Autodesk Inventor part; units mm, degrees
ref_plane "YZ Plane" through (0, 0, 0) normal (1, 0, 0) x (0, 1, 0)
ref_plane "XZ Plane" through (0, 0, 0) normal (0, 1, 0) x (-1, 0, 0)
ref_plane "XY Plane" through (0, 0, 0) normal (0, 0, 1) x (1, 0, 0)
sketch "スケッチ1" plane through (0, 0, 0) normal (0, 0, 1) x (1, 0, 0)
  circle A0 centre (0, 0) radius 1.5
  dimension "d0" = 3
extrude "押し出し1" add sketch "スケッチ1" along normal blind 6
sketch "スケッチ2" plane through (0, 0, 6) normal (0, 0, 1) x (1, 0, 0)
  circle A0 centre (0, 0) radius 1.5
  circle A1 centre (0, 0) radius 3
  dimension "d3" = 6
extrude "押し出し2" add sketch "スケッチ2" along normal blind 2 contours A0 | A1
fillet "フィレット1" radius 2 1 edges at (-3, 0, 8)
thread "ねじ1"
sketch "スケッチ3" plane through (0, 0, 0) normal (0, 0, -1) x (-1, 0, 0)
  circle A0 centre (0, 0) radius 1.5
extrude "押し出し3" add sketch "スケッチ3" along normal blind 9
sketch "スケッチ4" plane through (0, 0, 8) normal (0, 0, 1) x (1, 0, 0)
  line L0 (0.8191, 1.1885) -> (1.4388, -0.1151)
  line L1 (1.4388, -0.1151) -> (0.6197, -1.3036)
  line L2 (0.6197, -1.3036) -> (-0.8191, -1.1885)
  line L3 (-0.8191, -1.1885) -> (-1.4388, 0.1151)
  line L4 (-1.4388, 0.1151) -> (-0.6197, 1.3036)
  line L5 (-0.6197, 1.3036) -> (0.8191, 1.1885)
  point P0 (0, 0)
  point P1 (0, 0)
  dimension "d11" = 2.5
extrude "押し出し4" cut sketch "スケッチ4" against normal blind 1.3
properties part number "SB　15mmなべネジ" material "Steel, Mild"
The listing builds one solid part. Answer for the finished solid, in the listing's coordinates (mm). A direction names the side the tool comes from. Round coordinates to 2 decimals unless told otherwise and drop trailing zeros. Write each loop counter-clockwise with the first axis right and the second up, starting at its lowest first coordinate (ties: lowest second). Pieces come first, ordered by that corner, then holes. Notation, with made-up numbers: M -14.75,71 L -1.75,71 A16 ccw -1.75,89 Z; hole C 32.5,41 d10. An arc over 180 degrees is marked long. Write each question's results on one line, items separated by ' | '. Start each with the question number.
Item 1: A cutting plane is placed at A-A on z = -5. Write down the section's boundary in (x, y), and give its area (3 significant figures).
Item 2: Straight lines are drawn through the part: L1, parallel to X at y = -0.75, z = -5.75; L2, parallel to Z at x = 0.25, y = 1; L3, parallel to X at y = 0, z = 4.5. For each, find the intervals that lie inside material, in ascending order. Write a range as [from, to].
Item 3: Flat-ended cylindrical pins translate along their axes: pin 1 Ø1.5 at (x, y) = (2.5, -1.5) entering from +Z; pin 2 Ø0.8 at (x, y) = (0, -0.5) entering from +Z; pin 3 Ø2 at (y, z) = (-1.5, 6) entering from -X. Find the tip coordinate at first contact, or state that the pin passes through.
Item 4: For faces 1 (the face through (1.3, -1.3, 6)), 2 (the face through (0, 0, -9)), 3 (the face through (-1.125, -0.546, 7.351)), determine the directions among +Z, -Z, +X, -X, +Y, -Y from which every point of the face is accessible in a straight line to the end or side of a thin tool.
Check sheet entries:
1) outline: C 0,0 d3 | area: 7.07 mm²
2) L1: [-1.3, 1.3] | L2: [-9, 6.7] | L3: [-1.5, 1.5]
3) pin 1: z = 7.63 | pin 2: z = 6.7 | pin 3: x = -2.96
4) face 1: -Z | face 2: -Z, +X, -X, +Y, -Y | face 3: +Z
